Answer from the drawing. Dimensions are ordinates in mm from the lowest x, y and z of the part. A direction names the side the tool comes from. Round coordinates to 2 decimals unless told otherwise and drop trailing zeros. Loops run counter-clockwise (first coordinate to the right, second up) from the corner with the lowest first, then second, coordinate; pieces in that order, holes last. Notation, with made-up numbers: M 41.25,86.5 L 70.25,86.5 A35 cw 70.25,122.5 Z; hole C -19.5,42 d11. An arc over 180 degrees is marked long. Answer as a JSON object with one key per item and string values.
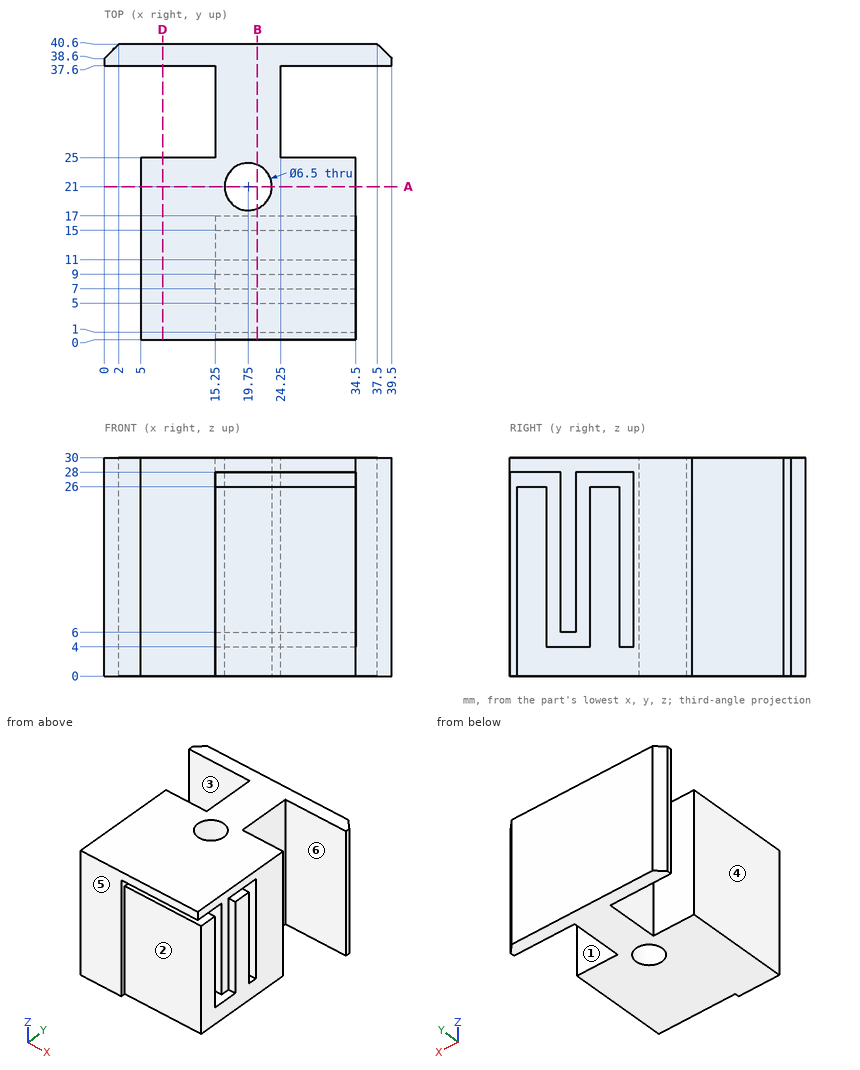
Item 1: The part is cut by section B-B (x = 21). Give the vertices of the cut face in (y, z).
Values follow:
{"outline": "M 0,28 L 7,28 L 7,6 L 9,6 L 9,28 L 17,28 L 17,4 L 15,4 L 15,26 L 11,26 L 11,4 L 5,4 L 5,26 L 1,26 L 1,0 L 18,0 L 18,30 L 0,30 Z; M 24,0 L 40.6,0 L 40.6,30 L 24,30 Z"}
Item 2: Which of the six approach directions +Z, -Z, +X, -X, +Y, -Y give full straight-line access (tool end or side, diameter ignored) to the marked faces 1, 2 and 3?
Values follow:
{"face 1": "+Z, -Z, +X", "face 2": "-Z, +X, -Y", "face 3": "+Z, -Z, -X"}
Item 3: Flat-ended cylindrical pins translate along their axes: P1, Ø5, axis at x = 20, z = 23.5, coming from the -Y side; P2, Ø4.5, axis at x = 8.5, z = 9.5, coming from the -Y side; P3, Ø1.5, axis at y = 23, z = 21, coming from the -X side; P4, Ø7.5, axis at y = 18.5, z = 11, coming from the +X side. Find the tip coordinate at first contact, or state that the pin passes through.
Values follow:
{"P1": "y = 1", "P2": "y = 0", "P3": "x = 5", "P4": "x = 34.5"}
Item 4: Straight lines are drawn through the part: line 1 (Y direction, x = 19.75, z = 10.5); line 2 (Y direction, x = 15.5, z = 19); line 3 (Y direction, x = 12, z = 28.75). For each, find the intervals that lie inside material, in ascending order.
Values follow:
{"line 1": "1 to 5, 7 to 9, 11 to 15, 17 to 17.75, 24.25 to 40.6", "line 2": "1 to 5, 7 to 9, 11 to 15, 17 to 40.6", "line 3": "0 to 25, 37.6 to 40.6"}
Item 5: The part is cut by section D-D (x = 8). Give the vertices of the cut face in (y, z).
Values follow:
{"outline": "M 0,0 L 25,0 L 25,30 L 0,30 Z; M 37.6,0 L 40.6,0 L 40.6,30 L 37.6,30 Z"}
Item 6: Determine the mould class of the marked faces 4, 5 and 6 for opening direction Y: released by +Y, released by -Y, zero draft, split by the parting line, or undercut.
Values follow:
{"face 4": "zero draft", "face 5": "released by -Y", "face 6": "undercut"}
Item 7: The part is cut by section A-A (y = 21). Give the vertices of the cut face in (x, z).
Values follow:
{"outline": "M 5,0 L 16.5,0 L 16.5,30 L 5,30 Z; M 23,0 L 34.5,0 L 34.5,30 L 23,30 Z"}
